Here's how the part is built. I have some questions about the finished solid (model axes, mm). Give positions to 0.01 mm unless a question says otherwise; leave off trailing zeros. Loops run counter-clockwise (first coordinate to the right, second up) from the corner with the lowest first, then second, coordinate; pieces in that order, holes last. Notation, with made-up numbers: M 65.25,-31 L 75.25,-31 A16 cw 75.25,0 Z; hole C 0.5,-19 d8. An arc over 180 degrees is marked long. Answer as CSV lines item,"result". Start each with the question number.
Item 1: Will this pin go through, and if not, where does the flat tip stop? P1, Ø1.1, axis at x = 16.59, z = -28.59, coming from the -Y side.
Item 2: I want a section at B-B on z = -20.5. List the corners of the cut face in (x, y) for me, plus the area to 3 significant figures.
Item 3: I want a section at A-A on x = -4.5. List the corners of the cut face in (y, z) for me.
Item 4: If I drill on line 1 along X through (y, z) = (0.9, 11.5); line 2 along Z through (x, y) = (-17, 2.4); line 3 along Z through (x, y) = (3.5, 1.95), over which ranges is the centre line in solid material (lowest first)? Write a range as from..to.
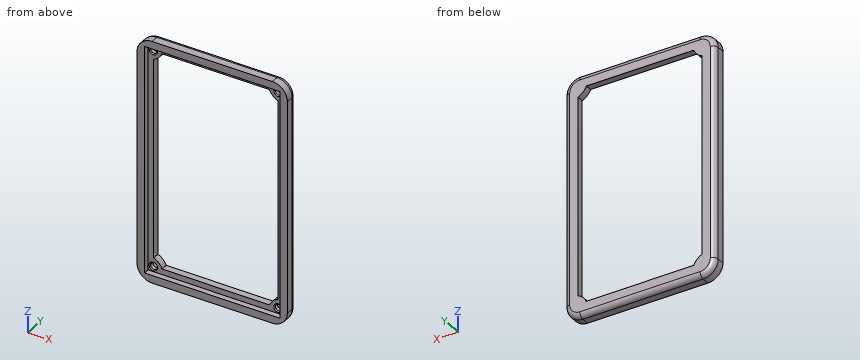
from build123d import *

# Parameters (mm, degrees)
SKETCH1_W                          = 40
SKETCH1_H                          = 64
SKETCH1_W_2                        = 36
SKETCH1_H_2                        = 60
BOSS_EXTRUDE1_DEPTH                = 3.3
SKETCH3_W                          = 36
SKETCH3_H                          = 60
BOSS_EXTRUDE2_DEPTH                = 1.8
FILLET1_R                          = 4
M2_2X0_45_TAPPED_HOLE1_D           = 1.75
M2_2X0_45_TAPPED_HOLE1_DEPTH       = 1.2
M2_2X0_45_TAPPED_HOLE1_CSINK_D     = 2.25
M2_2X0_45_TAPPED_HOLE1_CSINK_ANGLE = 90
M2_2X0_45_TAPPED_HOLE1_TIP         = 0.525753042
FILLET3_R                          = 1.3


with BuildPart() as part:
    # Sketch1 → Boss-Extrude1 (new body)
    with BuildSketch(Plane(origin=(0, 0, 0), x_dir=(1, 0, 0), z_dir=(0, 1, 0))):
        Rectangle(SKETCH1_W, SKETCH1_H)
        Rectangle(SKETCH1_W_2, SKETCH1_H_2, mode=Mode.SUBTRACT)
    extrude(amount=BOSS_EXTRUDE1_DEPTH)

    # Sketch3 → Boss-Extrude2 (add)
    with BuildSketch(Plane(origin=(0, 3.3, 0), x_dir=(1, 0, 0), z_dir=(0, 1, 0))):
        Rectangle(SKETCH3_W, SKETCH3_H)
        with BuildLine():
            ThreePointArc((14.291900756, 28.5), (15.171572875, 27.171572875), (16.5, 26.291900756))
            Line((16.5, 26.291900756), (16.5, -26.291900756))
            ThreePointArc((16.5, -26.291900756), (15.171572875, -27.171572875), (14.291900756, -28.5))
            Line((14.291900756, -28.5), (-14.291900756, -28.5))
            ThreePointArc((-14.291900756, -28.5), (-15.171572875, -27.171572875), (-16.5, -26.291900756))
            Line((-16.5, -26.291900756), (-16.5, 26.291900756))
            ThreePointArc((-16.5, 26.291900756), (-15.171572875, 27.171572875), (-14.291900756, 28.5))
            Line((-14.291900756, 28.5), (14.291900756, 28.5))
        make_face(mode=Mode.SUBTRACT)
    extrude(amount=-BOSS_EXTRUDE2_DEPTH)

    # Fillet1
    fillet1_edges = [part.edges().sort_by_distance(p)[0] for p in [
        (-20, 1.65, -32),
        (20, 1.65, -32),
        (20, 1.65, 32),
        (-20, 1.65, 32),
    ]]
    fillet(fillet1_edges, radius=FILLET1_R)

    # M2.2x0.45 Tapped Hole1
    with Locations(Plane.XZ.offset(-1.5)):
        with Locations((-16.585786438, 28.585786438), (16.585786438, 28.585786438), (-16.585786438, -28.585786438), (16.585786438, -28.585786438)):
            CounterSinkHole(M2_2X0_45_TAPPED_HOLE1_D / 2, M2_2X0_45_TAPPED_HOLE1_CSINK_D / 2, depth=M2_2X0_45_TAPPED_HOLE1_DEPTH, counter_sink_angle=M2_2X0_45_TAPPED_HOLE1_CSINK_ANGLE)
            with Locations((0, 0, -(M2_2X0_45_TAPPED_HOLE1_DEPTH + M2_2X0_45_TAPPED_HOLE1_TIP / 2))):  # 118° drill point
                Cone(0, M2_2X0_45_TAPPED_HOLE1_D / 2, M2_2X0_45_TAPPED_HOLE1_TIP, mode=Mode.SUBTRACT)

    # Fillet3
    fillet3_edges = [part.edges().sort_by_distance(p)[0] for p in [
        (0, 3.3, -32),
        (20, 3.3, 0),
        (-20, 3.3, 0),
        (0, 3.3, 32),
        (-18.828427125, 3.3, 30.828427125),
        (18.828427125, 3.3, 30.828427125),
        (-18.828427125, 3.3, -30.828427125),
        (18.828427125, 3.3, -30.828427125),
    ]]
    fillet(fillet3_edges, radius=FILLET3_R)


solid = part.part
Result:
1,P1,"y = 2.89"
2,outline,"M -20,0 L -18,0 L -18,1.5 L -16.5,1.5 L -16.5,3.3 L -18.7,3.3 A1.3 ccw -20,2 Z; M 16.5,1.5 L 18,1.5 L 18,0 L 20,0 L 20,2 A1.3 ccw 18.7,3.3 L 16.5,3.3 Z"
2,area,"17.9 mm^2"
3,outline,"M 0,-32 L 2,-32 A1.3 ccw 3.3,-30.7 L 3.3,-28.5 L 1.5,-28.5 L 1.5,-30 L 0,-30 Z; M 0,30 L 1.5,30 L 1.5,28.5 L 3.3,28.5 L 3.3,30.7 A1.3 ccw 2,32 L 0,32 Z"
4,line 1,"-20..-18, 18..20"
4,line 2,"-31.81..-29.36, -27.82..27.82, 29.36..31.81"
4,line 3,"-32..-28.5, 28.5..32"
